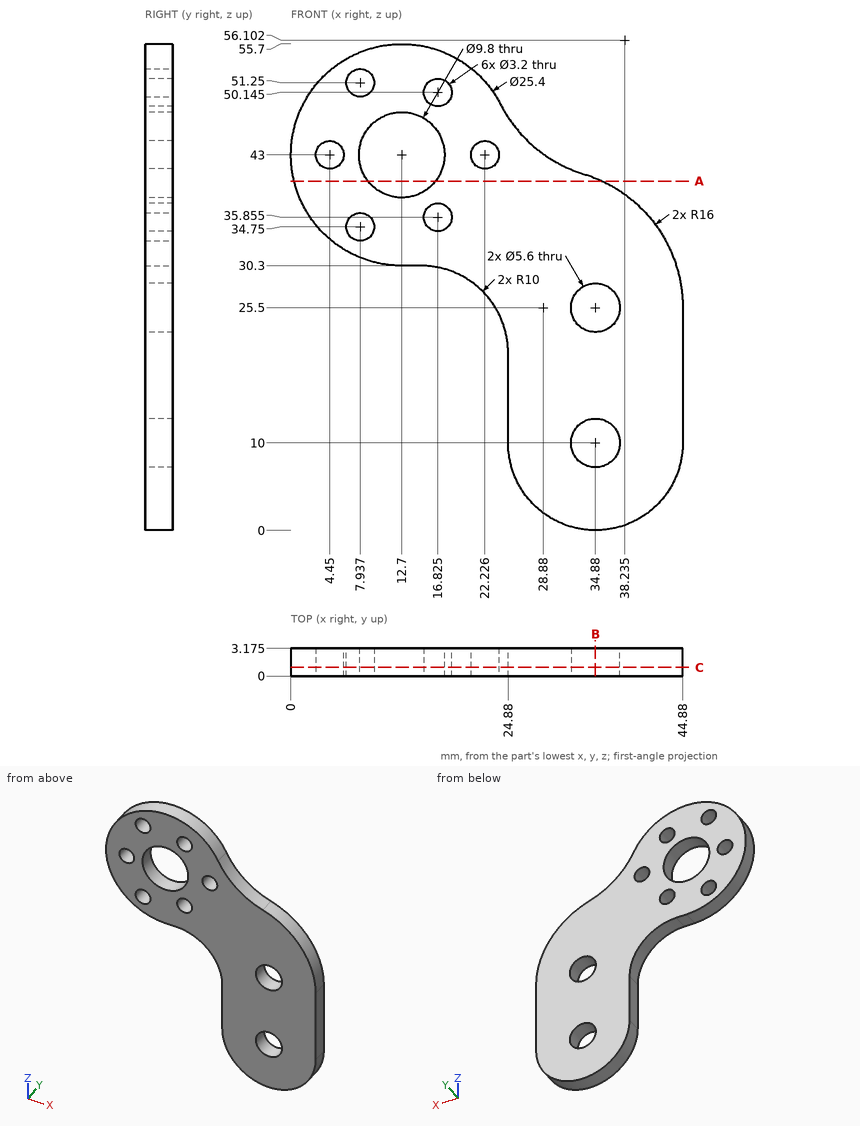
Here's the drawing with two shaded views (mm, measured from the low corner). I have some questions. Coordinates: 2 decimals unless noted, no trailing zeros. Order: outer loops, then holes, each group sorted by start corner. A loop starts at its lowest first (then second) coordinate and runs counter-clockwise, first axis right, second up. Notation, with made-up numbers: (-1, 75.25) - (5, 75.25) arc R21 cw to (5, 108.25) - close; hole circle Ø3 at (86, 40). An arc over 180 degrees is marked (long way). Answer in a Markdown table with one row per item.
1. Suppose I cut it at A-A (z = 40). Please give me the cut outline in (x, y) (1 decimal).
Reply:
| item | result |
|---|---|
| outline | (0.4, 0) - (8.8, 0) - (8.8, 3.2) - (0.4, 3.2) - close; (16.6, 0) - (35.6, 0) - (35.6, 3.2) - (16.6, 3.2) - close |
2. If I drill on line 1 along X through (y, z) = (1.65, 10); line 2 along X through (y, z) = (2.1, 51.25) (1 decimal); line 3 along Z through (x, y) = (34.88, 1.35), over which ranges is the centre line in solid material (lowest first)?
Reply:
| item | result |
|---|---|
| line 1 | x = 24.88 to 32.08, 37.68 to 44.88 |
| line 2 | x = 3 to 6.3, 9.5 to 15.7, 18 to 22.4 |
| line 3 | z = 0 to 7.2, 12.8 to 22.7, 28.3 to 40.33 |
3. Suppose I cut it at C-C (y = 1). Give the number of separate pieces and of enclosed holes in the cut face, and give its area (3 significant figures).
Reply:
| item | result |
|---|---|
| separate pieces | 1 |
| enclosed holes | 9 |
| area | 1,130 mm^2 |
4. Suppose I cut it at B-B (x = 34.88). Please give me the cut outline in (y, z) (1 decimal), and give its area (3 significant figures).
Reply:
| item | result |
|---|---|
| outline | (0, 0) - (3.2, 0) - (3.2, 7.2) - (0, 7.2) - close; (0, 12.8) - (3.2, 12.8) - (3.2, 22.7) - (0, 22.7) - close; (0, 28.3) - (3.2, 28.3) - (3.2, 40.3) - (0, 40.3) - close |
| area | 92.5 mm^2 |
5. For pin 1 (1.1 mm diameter, centred on x = 14, y = 1.5, fed in from -Z); pin 2 (6.5 mm diameter, centred on x = 34.88, z = 10, fed in from -Y); pin 3 (9 mm diameter, centred on x = 12.7, z = 43, fed in from +Y), each with a flat end and sliding along its axis, tell me the tip position at first contact or that it passes through.
Reply:
| item | result |
|---|---|
| pin 1 | stops at z = 30.3 |
| pin 2 | stops at y = 0 |
| pin 3 | passes through |
